Work out the finished part from the listing and answer in its coordinate system (mm). Coordinates: 2 decimals unless noted, no trailing zeros. Order: outer loops, then holes, each group sorted by start corner. A loop starts at its lowest first (then second) coordinate and runs counter-clockwise, first axis right, second up. Notation, with made-up numbers: M 78.5,51 L 114.5,51 A16 cw 114.5,69 Z; hole C -4.5,15.25 d2. An arc over 180 degrees is marked long. Use a Markdown table: item, result.
from build123d import *

# Parameters (mm, degrees)
SKETCH010_R  = 3
SKETCH010_W  = 2
SKETCH010_H  = 5
PAD010_DEPTH = 5


with BuildPart() as part:
    # Sketch010 → Pad010 (new body)
    with BuildSketch(Plane.XY):
        Polygon((-10, 160.1), (-20, 160.1), (-47.2, -130.1), (-33.6, -130.1), (-33.6, -155.2), (-13.4, -155.2), (-13.4, -130.1), (13.4, -130.1), (13.4, -155.2), (33.6, -155.2), (33.6, -130.1), (47.2, -130.1), (20, 160.1), (10, 160.1), (10, 185.1), (-10, 185.1), align=None)
        with Locations((0, -100)):
            Circle(SKETCH010_R, mode=Mode.SUBTRACT)
        with Locations((0, 100)):
            Circle(SKETCH010_R, mode=Mode.SUBTRACT)
        with Locations((-10, -80)):
            Rectangle(SKETCH010_W, SKETCH010_H, mode=Mode.SUBTRACT)
        with Locations((10, -80)):
            Rectangle(SKETCH010_W, SKETCH010_H, mode=Mode.SUBTRACT)
        with Locations((-10, -120)):
            Rectangle(SKETCH010_W, SKETCH010_H, mode=Mode.SUBTRACT)
        with Locations((10, -120)):
            Rectangle(SKETCH010_W, SKETCH010_H, mode=Mode.SUBTRACT)
        with Locations((-10, 120)):
            Rectangle(SKETCH010_W, SKETCH010_H, mode=Mode.SUBTRACT)
        with Locations((10, 120)):
            Rectangle(SKETCH010_W, SKETCH010_H, mode=Mode.SUBTRACT)
        with Locations((-10, 80)):
            Rectangle(SKETCH010_W, SKETCH010_H, mode=Mode.SUBTRACT)
        with Locations((10, 80)):
            Rectangle(SKETCH010_W, SKETCH010_H, mode=Mode.SUBTRACT)
    extrude(amount=PAD010_DEPTH)


solid = part.part
1. Section D-D on y = 100 is taken. Determine the outline of the cut face in (x, z), then the cut area to 3 significant figures.
Answers below:
| item | result |
|---|---|
| outline | M -25.63,0 L -3,0 L -3,5 L -25.63,5 Z; M 3,0 L 25.63,0 L 25.63,5 L 3,5 Z |
| area | 226 mm² |
2. Flat-ended cylindrical pins translate along their axes: P1, Ø0.6, axis at x = 10.5, z = 2.5, coming from the +Y side; P2, Ø1.5, axis at y = -80, z = 1.5, coming from the -X side; P3, Ø1, axis at x = -9.5, z = 2.5, coming from the -Y side; P4, Ø5, axis at x = -19, y = -15.5, coming from the -Z side. Find the tip coordinate at first contact, or state that the pin passes through.
Answers below:
| item | result |
|---|---|
| P1 | y = 160.1 |
| P2 | x = -42.57 |
| P3 | y = -130.1 |
| P4 | z = 0 |
3. Find the intervals of material crossed by probe 1 along Y at (x, z) = (0, 1.15); probe 2 along X at (y, z) = (-137.5, 4.55); probe 3 along Y at (x, z) = (16.5, 3.2), in increasing order.
Answers below:
| item | result |
|---|---|
| probe 1 | -130.1 to -103, -97 to 97, 103 to 185.1 |
| probe 2 | -33.6 to -13.4, 13.4 to 33.6 |
| probe 3 | -155.2 to 160.1 |
4. Section A-A on x = 0 is taken. Determine the outline of the cut face in (y, z).
Answers below:
| item | result |
|---|---|
| outline | M -130.1,0 L -103,0 L -103,5 L -130.1,5 Z; M -97,0 L 97,0 L 97,5 L -97,5 Z; M 103,0 L 185.1,0 L 185.1,5 L 103,5 Z |
5. Section B-B on y = -100 is taken. Determine the outline of the cut face in (x, z), then the cut area to 3 significant figures.
Answers below:
| item | result |
|---|---|
| outline | M -44.38,0 L -3,0 L -3,5 L -44.38,5 Z; M 3,0 L 44.38,0 L 44.38,5 L 3,5 Z |
| area | 414 mm² |
6. For a pull along X with two mould halves and no side action, classify faces 1 (the face through (-1, -20, 0)), 2 (the face through (33.79, 12.97, 2.46)), 3 (the face through (-0.65, 97.07, 2.46)), 4 (the face through (-0.65, -102.93, 2.46)) as +X half, -X half, draft (parallel to the pull), parting line (faces both ways), or undercut.
Answers below:
| item | result |
|---|---|
| face 1 | draft |
| face 2 | +X half |
| face 3 | undercut |
| face 4 | undercut |
7. Section C-C on z = 2.7 is taken. Give the number of separate pieces and of enclosed holes in the cut face, then the cut area to 3 significant figures.
Answers below:
| item | result |
|---|---|
| separate pieces | 1 |
| enclosed holes | 10 |
| area | 20,900 mm² |
